Work out the finished part from the listing and answer in its coordinate system (mm). A direction names the side the tool comes from. Coordinates: 2 decimals unless noted, no trailing zeros. Order: outer loops, then holes, each group sorted by start corner. A loop starts at its lowest first (then second) coordinate and runs counter-clockwise, first axis right, second up. Notation, with made-up numbers: M 73.5,71 L 84.5,71 A11 cw 84.5,85 Z; hole C 49.5,17.5 d8. An arc over 180 degrees is marked long. Write item = value, one per line. Start each with the question number.
Q1. Straight lines are drawn through the part: line 1 along Z through (x, y) = (20, 1) (3 decimals); line 2 along X through (y, z) = (31, 17.5). For each, find the intervals that lie inside material, in ascending order.
Q2. A tool of negligible diameter and unlimited length cuts with its end or side. For faces 4 (the flat face through (14, 1.5, 11)), 5 (the cylindrical face through (0.34, 0.32, 10.92)), from which of +Z, -Z, +X, -X, +Y, -Y can it reach the whole face along a straight path? Write none if from no direction.
Q3. Find section B-B on y = 30. Give the vertices of the cut face in (x, z) (3 decimals).
Q4. Each of these flat-tipped pins is pushed along its axis until it touches: P1, Ø3, axis at x = 20, z = 4.325, coming from the -Y side; P2, Ø5, axis at y = 17, z = 6, coming from the +X side. Where does it stop, or does it pass through?
Q5. Determine the mould class of faces 1 (the cylindrical face through (18.41, 0.76, 5.54)), 2 (the flat face through (1.5, 19, 11)), 3 (the flat face through (13, 0, 11)) for opening direction X: released by +X, released by -X, zero draft, split by the parting line, or undercut.
Q6. Find section A-A on x = 20. Give the vertices of the cut face in (y, z) (3 decimals), and give its area (3 significant figures).
Q7. Find section C-C on z = 11.75. Give the vertices of the cut face in (x, y).
Q8. Find section D-D on x = 6.5. Give the vertices of the cut face in (y, z), and give its area (3 significant figures).
```python
from build123d import *

# Parameters (mm, degrees)
BOSS_EXTRU_1_DEPTH      = 22.15
ESQUISSE2_R             = 2
ENL_V_MAT_EXTRU_1_DEPTH = 2.5
ESQUISSE3_R             = 1
ENL_V_MAT_EXTRU_2_DEPTH = 2.5


with BuildPart() as part:
    # Esquisse1 → Boss.-Extru.1 (new body)
    with BuildSketch(Plane.XY):
        with BuildLine():
            Line((0, 1.122291019), (0, 34))
            Line((0, 34), (1.5, 34))
            Line((1.5, 34), (1.5, 2.622291019))
            ThreePointArc((1.5, 2.622291019), (1.828711429, 1.828711429), (2.622291019, 1.5))
            Line((2.622291019, 1.5), (25, 1.5))
            Line((25, 1.5), (25, 0))
            Line((25, 0), (1.122291019, 0))
            ThreePointArc((1.122291019, 0), (0.328711429, 0.328711429), (0, 1.122291019))
        make_face()
    extrude(amount=BOSS_EXTRU_1_DEPTH)

    # Esquisse2 → Enlèv. mat.-Extru.1 (cut, through all)
    with BuildSketch(Plane(origin=(0, 1.5, 0), x_dir=(1, 0, 0), z_dir=(0, 1, 0))):
        with Locations((20, -4.325)):
            Circle(ESQUISSE2_R)
        with Locations((20, -17.825)):
            Circle(ESQUISSE2_R)
    extrude(amount=-ENL_V_MAT_EXTRU_1_DEPTH, mode=Mode.SUBTRACT)

    # Esquisse3 → Enlèv. mat.-Extru.2 (cut, through all)
    with BuildSketch(Plane(origin=(1.5, 0, 0), x_dir=(0, 0, -1), z_dir=(1, 0, 0))):
        with Locations((-16.075, 30)):
            Circle(ESQUISSE3_R)
        with Locations((-6.075, 30)):
            Circle(ESQUISSE3_R)
    extrude(amount=-ENL_V_MAT_EXTRU_2_DEPTH, mode=Mode.SUBTRACT)


solid = part.part
```
Findings below:
q1.line_1 = 0 to 2.325, 6.325 to 15.825, 19.825 to 22.15
q1.line_2 = 0 to 1.5
q2.face_4 = +Z, -Z, +X, +Y
q2.face_5 = +Z, -Z, -X, -Y
q3.outline = M 0,0 L 1.5,0 L 1.5,5.075 L 0,5.075 Z; M 0,7.075 L 1.5,7.075 L 1.5,15.075 L 0,15.075 Z; M 0,17.075 L 1.5,17.075 L 1.5,22.15 L 0,22.15 Z
q4.P1 = through
q4.P2 = 1.5
q5.face_1 = undercut
q5.face_2 = released by +X
q5.face_3 = zero draft
q6.outline = M 0,0 L 1.5,0 L 1.5,2.325 L 0,2.325 Z; M 0,6.325 L 1.5,6.325 L 1.5,15.825 L 0,15.825 Z; M 0,19.825 L 1.5,19.825 L 1.5,22.15 L 0,22.15 Z
q6.area = 21.2 mm^2
q7.outline = M 0,1.12 A1.12 ccw 1.12,0 L 25,0 L 25,1.5 L 2.62,1.5 A1.12 cw 1.5,2.62 L 1.5,34 L 0,34 Z
q8.outline = M 0,0 L 1.5,0 L 1.5,22.15 L 0,22.15 Z
q8.area = 33.2 mm^2
